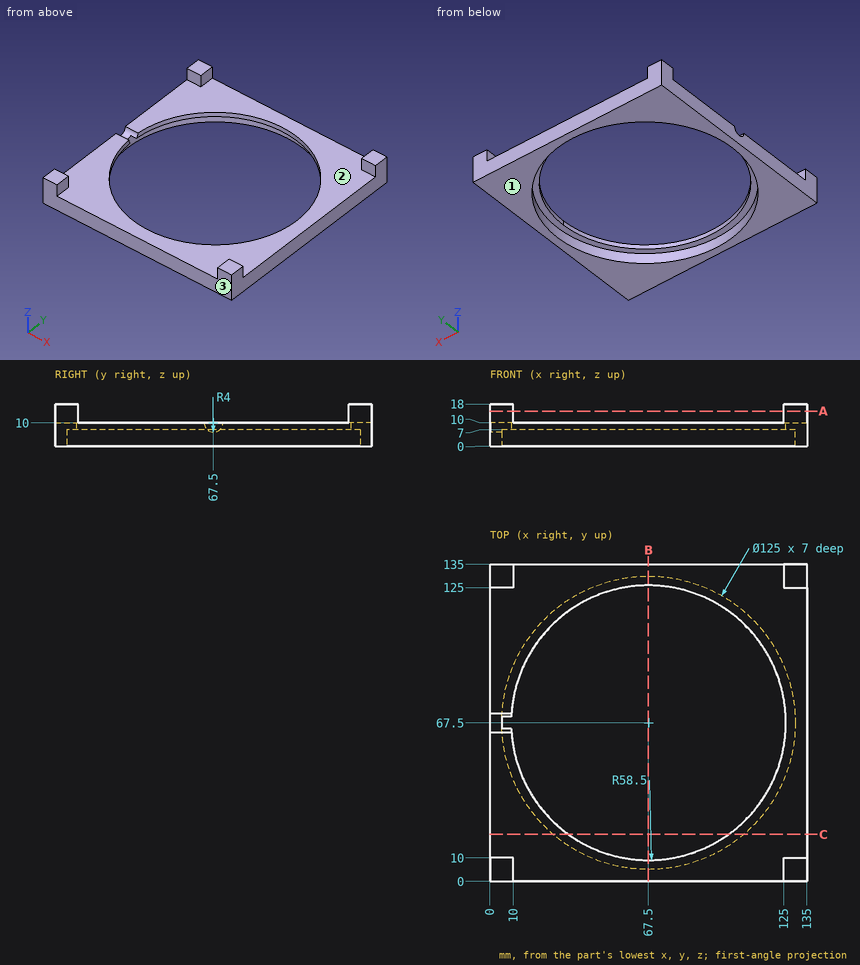
Here's the drawing with two shaded views (mm, measured from the low corner). I have some questions. Give positions to 0.01 mm unless a question says otherwise; leave off trailing zeros. Loops run counter-clockwise (first coordinate to the right, second up) from the corner with the lowest first, then second, coordinate; pieces in that order, holes last. Notation, with made-up numbers: M 6.25,62.5 L 51.25,62.5 A25 cw 51.25,98.5 Z; hole C 75,-13.75 d4. An arc over 180 degrees is marked long. Use one line per item in the form item = value. Start each with the question number.
(1) I want a section at B-B, the plane x = 67.5. Write out the boundary of the cut face in (y, z), and give its area (3 significant figures).
(2) Please list where these lines run through material, in increasing order: line 1 (Y direction, x = 67.5, z = 5); line 2 (Z direction, x = 124, y = 6).
(3) I want a section at A-A, the plane z = 15. Write out the boundary of the cut face in (x, y), and give its area (3 significant figures).
(4) I'm going to push flat-ended pins straight in: P1, Ø1, axis at x = 20, y = 113.5, coming from the +Z side; P2, Ø6, axis at y = 49.5, z = 11, coming from the -X side. Where does each tip first touch, or does it pass through?
(5) I want a section at C-C, the plane y = 20. Write out the boundary of the cut face in (x, z), and give its area (3 significant figures).
(6) Thinking about a two-plate mould opening in Y: for the marked faces 1, 2 and 3, which applies, released by +Y, released by -Y, zero draft, split by the parting line, or undercut?
Worked out:
q1.outline = M 0,0 L 5,0 L 5,7 L 9,7 L 9,10 L 0,10 Z; M 126,7 L 130,7 L 130,0 L 135,0 L 135,10 L 126,10 Z
q1.area = 124 mm²
q2.line_1 = 0 to 5, 130 to 135
q2.line_2 = 0 to 10
q3.outline = M 0,0 L 10,0 L 10,10 L 0,10 Z; M 0,125 L 10,125 L 10,135 L 0,135 Z; M 125,0 L 135,0 L 135,10 L 125,10 Z; M 125,125 L 135,125 L 135,135 L 125,135 Z
q3.area = 400 mm²
q4.P1 = 10
q4.P2 = 0
q5.outline = M 0,0 L 26.88,0 L 26.88,7 L 33.35,7 L 33.35,10 L 0,10 Z; M 101.65,7 L 108.12,7 L 108.12,0 L 135,0 L 135,10 L 101.65,10 Z
q5.area = 576 mm²
q6.face_1 = zero draft
q6.face_2 = undercut
q6.face_3 = released by -Y
